For this review, take the finished solid that the model builds, in its own axes (mm). A direction names the side the tool comes from. Round coordinates to 2 decimals unless told otherwise and drop trailing zeros. Write each loop counter-clockwise with the first axis right and the second up, starting at its lowest first coordinate (ties: lowest second). Pieces come first, ordered by that corner, then holes. Notation, with made-up numbers: (77, 69.25) -> (115, 69.25) arc R3 cw to (115, 73.25) -> close; hole circle Ø7 at (50.5, 16.25). An arc over 180 degrees is marked (long way). Write each question's results on one line, items separated by ' | '. Start each with the question number.
Item 1: Add section A-A (y = 3.75). State the section outline as (x, z) points, plus the area to 3 significant figures.
Item 2: Clearance check with flat-ended pins moving along their axes: pin 1 (1.5 mm diameter, centred on x = -1.5, y = 1.5, fed in from -Z); pin 2 (1 mm diameter, centred on x = -5, y = 2, fed in from -Z); pin 3 (10 mm diameter, centred on x = 6, z = -2, fed in from +Y); pin 4 (1.5 mm diameter, centred on x = 7, z = 1.5, fed in from -Y). State where each tip first meets the part, or that it passes through.
Item 3: To check wall thickness, follow line 1 along X through (y, z) = (3.15, 0); line 2 along X through (y, z) = (4.65, 0); line 3 along Z through (x, y) = (-1, 0.5). State the ranges of each line that lie inside material, in increasing order.
Item 4: Tool access review of faces 3 (the cylindrical face through (3.16, 5.01, 7.89)), 4 (the cylindrical face through (8.11, 1.25, -2.55)), 5 (the cylindrical face through (2.703, 1.993, 8.584)): name each direction out of +Z, -Z, +X, -X, +Y, -Y from which nothing blocks a thin tool from reaching the whole face with its end or side.
Item 5: The part is to be moulded in two halves that separate along X. For faces 1 (the cylindrical face through (8.11, 2.75, -2.55)), 2 (the cylindrical face through (-7.81, 3.04, -1.73)), say which applies: +X half, -X half, draft (parallel to the pull), parting line (faces both ways), or undercut.
Item 6: Add section B-B (y = 5). State the section outline as (x, z) points, plus the area to 3 significant figures.
from build123d import *

# Parameters (mm, degrees)
SKETCH_1_R          = 9
EXTRUDE_1_DEPTH     = 4.5
SKETCH_2_W          = 1
SKETCH_2_H          = 0.5
SKETCH_4_R          = 8
CUT_EXTRUDE_1_DEPTH = 4.5
EXTRUDE_START       = 1.5
SKETCH_6_R          = 8.5
SKETCH_6_R_2        = 8
EXTRUDE_3_DEPTH     = 1.5


with BuildPart() as part:
    # 草图1 → 凸台-拉伸1 (new body)
    with BuildSketch(Plane(origin=(0, 0, 0), x_dir=(1, 0, 0), z_dir=(0, 1, 0))):
        with Locations(Location((0, 0, 0), (0, 0, 270))):
            Circle(SKETCH_1_R)
    extrude(amount=EXTRUDE_1_DEPTH)

    # 切除-扫描1: sweep along a path in 草图3
    with BuildLine(Plane(origin=(0, 4.5, 0), x_dir=(1, 0, 0), z_dir=(0, 1, 0))) as sweep_1_path:
        CenterArc((0, 0), 9, 0, 360)
    # 草图2 → 切除-扫描1 (sweep, cut)
    with BuildSketch(Plane(origin=(0, 0, 0), x_dir=(0, 0, -1), z_dir=(1, 0, 0))):
        with Locations((-9, 4.25)):
            Rectangle(SKETCH_2_W, SKETCH_2_H)
        with Locations((-9, 2.75)):
            Rectangle(SKETCH_2_W, SKETCH_2_H)
        with Locations((-9, 1.25)):
            Rectangle(SKETCH_2_W, SKETCH_2_H)
    sweep(path=sweep_1_path.line, mode=Mode.SUBTRACT)

    # 草图4 → 切除-拉伸1 (cut)
    with BuildSketch(Plane(origin=(0, 4.5, 0), x_dir=(1, 0, 0), z_dir=(0, 1, 0))):
        with Locations(Location((0, 0, 0), (0, 0, 270))):
            Circle(SKETCH_4_R)
    extrude(amount=-CUT_EXTRUDE_1_DEPTH, mode=Mode.SUBTRACT)

    # 草图6 → 凸台-拉伸3 (add)
    with BuildSketch(Plane(origin=(0, 4.5, 0), x_dir=(1, 0, 0), z_dir=(0, 1, 0)).offset(EXTRUDE_START)):
        with Locations(Location((0, 0, 0), (0, 0, 270))):
            Circle(SKETCH_6_R)
        with Locations(Location((0, 0, 0), (0, 0, 270))):
            Circle(SKETCH_6_R_2, mode=Mode.SUBTRACT)
    extrude(amount=-EXTRUDE_3_DEPTH)


solid = part.part
Responses:
1) outline: circle Ø18 at (0, 0); hole circle Ø16 at (0, 0) | area: 53.4 mm^2
2) pin 1: stops at z = -8.97 | pin 2: stops at z = -7.79 | pin 3: stops at y = 6 | pin 4: passes through
3) line 1: x = -9 to -8, 8 to 9 | line 2: x = -8.5 to -8, 8 to 8.5 | line 3: z = -8.94 to -7.94, 7.94 to 8.94
4) face 3: +Y | face 4: none | face 5: +Y, -Y
5) face 1: parting line | face 2: undercut
6) outline: circle Ø17 at (0, 0); hole circle Ø16 at (0, 0) | area: 25.9 mm^2
